Read the model definition and answer for the solid it produces. Units are mm, in the model's axes. A direction names the side the tool comes from. Give positions to 0.01 mm unless a question says otherwise; leave off trailing zeros. Loops run counter-clockwise (first coordinate to the right, second up) from the corner with the lowest first, then second, coordinate; pieces in that order, holes last. Notation, with made-up numbers: (-7.5, 6.25) - (27.5, 6.25) arc R21 ccw to (27.5, 24.25) - close; hole circle Ø5 at (9, -28.5). An arc over 180 degrees is marked (long way). Use a Markdown table: item, result. Add a question column.
Item 1: A cutting plane is placed at D-D (y = -20.5). Determine the outline of the cut face in (x, z), plus the area to 3 significant figures.
Item 2: Which of the six approach directions +Z, -Z, +X, -X, +Y, -Y give full straight-line access (tool end or side, diameter ignored) to faces 1 (the face through (0, 5, -0.75)), 2 (the face through (-0.27, -29.98, -1.22)), 3 (the face through (0, -7.1, 1.5)), 4 (the face through (0, 5.954, 0))?
Item 3: Each of these flat-tipped pins is pushed along its axis until it touches: P1, Ø1.1, axis at x = 0.5, y = 5.5, coming from the -Z side; P2, Ø1.5, axis at y = -17, z = -1, coming from the -X side. Where does it stop, or does it pass through?
Item 4: A cutting plane is placed at C-C (y = 0.5). Determine the outline of the cut face in (x, z), plus the area to 3 significant figures.
Item 5: A cutting plane is placed at B-B (z = 0). Determine the outline of the cut face in (x, y).
Item 6: A cutting plane is placed at A-A (x = 0). Determine the outline of the cut face in (y, z).
Item 7: Consider probe 1 along Y at (x, z) = (1.1, -1.35); probe 2 along Y at (x, z) = (1.4, 0.1); probe 3 along X at (y, z) = (-2, 1.1). Determine where each line is inside the solid, lowest interval first. Write a range as [from, to].
from build123d import *

# Parameters (mm, degrees)
CUT_EXTRUDE_2_DEPTH = 23.35
CUT_EXTRUDE_3_DEPTH = 1.4


with BuildPart() as part:
    # 草图1 → 旋转2 (revolve)
    with BuildSketch(Plane.XY):
        Polygon((1.25, 5.954469818), (0, 5.954469818), (0, -30.845530182), (1.25, -30.845530182), (1.25, -29.145530182), (1.9, -29.145530182), (1.9, -17.395530182), (1.5, -17.395530182), (1.5, 2.854469818), (1.25, 2.854469818), align=None)
    revolve(axis=Axis((0, 5.954469818, 0), (0, -1, 0)))

    # 草图4 → 切除-拉伸2 (cut)
    with BuildSketch(Plane(origin=(0, 5.954469818, 0), x_dir=(1, 0, 0), z_dir=(0, 1, 0))):
        with BuildLine():
            Line((-1.118033989, 1), (1.118033989, 1))
            ThreePointArc((1.118033989, 1), (0, 1.5), (-1.118033989, 1))
        make_face()
    extrude(amount=-CUT_EXTRUDE_2_DEPTH, mode=Mode.SUBTRACT)

    # 草图5 → 切除-拉伸3 (cut)
    with BuildSketch(Plane(origin=(0, 5.954469818, 0), x_dir=(1, 0, 0), z_dir=(0, 1, 0))):
        with BuildLine():
            Line((-1, 0.75), (1, 0.75))
            ThreePointArc((1, 0.75), (0, 1.25), (-1, 0.75))
        make_face()
    extrude(amount=-CUT_EXTRUDE_3_DEPTH, mode=Mode.SUBTRACT)


solid = part.part
Geometry says:
| question | item | result |
|---|---|---|
| 1 | outline | circle Ø3.8 at (0, 0) |
| 1 | area | 11.3 mm² |
| 2 | face 1 | -Z, +X, -X, +Y |
| 2 | face 2 | -Y |
| 2 | face 3 | +Y |
| 2 | face 4 | +Z, -Z, +X, -X, +Y |
| 3 | P1 | z = -0.75 |
| 3 | P2 | x = -1.87 |
| 4 | outline | (-1.12, -1) - (1.12, -1) arc R1.5 ccw (long way) to start |
| 4 | area | 6.29 mm² |
| 5 | outline | (-1.9, -29.15) - (-1.25, -29.15) - (-1.25, -30.85) - (1.25, -30.85) - (1.25, -29.15) - (1.9, -29.15) - (1.9, -17.4) - (1.5, -17.4) - (1.5, 2.85) - (1.25, 2.85) - (1.25, 5.95) - (-1.25, 5.95) - (-1.25, 2.85) - (-1.5, 2.85) - (-1.5, -17.4) - (-1.9, -17.4) - close |
| 6 | outline | (-30.85, -1.25) - (-29.15, -1.25) - (-29.15, -1.9) - (-17.4, -1.9) - (-17.4, -1) - (4.55, -1) - (4.55, -0.75) - (5.95, -0.75) - (5.95, 1.25) - (2.85, 1.25) - (2.85, 1.5) - (-17.4, 1.5) - (-17.4, 1.9) - (-29.15, 1.9) - (-29.15, 1.25) - (-30.85, 1.25) - close |
| 7 | probe 1 | [-29.15, -17.4] |
| 7 | probe 2 | [-29.15, 2.85] |
| 7 | probe 3 | [-1.02, 1.02] |
